Could you check a few things on this drawing? It's one solid part, dimensions in mm from its lowest x, y, z. A direction names the side the tool comes from. Round coordinates to 2 decimals unless told otherwise and drop trailing zeros. Loops run counter-clockwise (first coordinate to the right, second up) from the corner with the lowest first, then second, coordinate; pieces in that order, holes last. Notation, with made-up numbers: M 29.5,-14 L 76.5,-14 A14 ccw 76.5,12 Z; hole C 62,24 d3. An arc over 180 degrees is marked long. Answer as a JSON object with one key per item and string values.
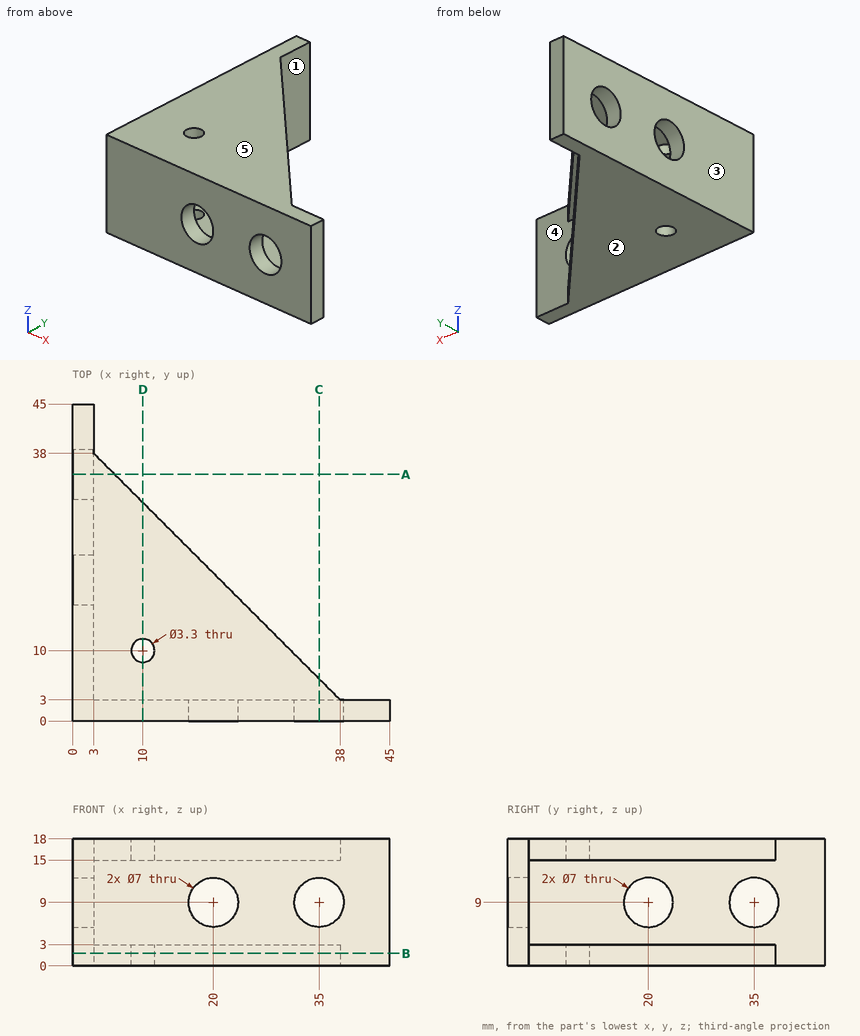
Item 1: Please list where these lines run through material, in increasing order: probe 1 along X at (y, z) = (1.9, 9); probe 2 along Z at (x, y) = (33, 4); probe 3 along Z at (x, y) = (1, 35). Write a range as from..to.
Resolved:
{"probe 1": "0..16.5, 23.5..31.5, 38.5..45", "probe 2": "0..3, 15..18", "probe 3": "0..5.5, 12.5..18"}
Item 2: I'm going to push flat-ended pins straight in: pin 1 Ø3 at (x, z) = (29, 11) entering from +Y; pin 2 Ø5 at (y, z) = (11.5, 2.5) entering from +X. Where does each tip first touch, or does it pass through?
Resolved:
{"pin 1": "y = 3", "pin 2": "x = 32"}
Item 3: I want a section at B-B, the plane z = 1.75. Please give me the cut outline in (x, y).
Resolved:
{"outline": "M 0,0 L 45,0 L 45,3 L 38,3 L 3,38 L 3,45 L 0,45 Z; hole C 10,10 d3.3"}
Item 4: I want a section at A-A, the plane y = 35. Please give me the cut outline in (x, z), then the cut area to 3 significant figures.
Resolved:
{"outline": "M 0,0 L 6,0 L 6,3 L 3,3 L 3,5.5 L 0,5.5 Z; M 0,12.5 L 3,12.5 L 3,15 L 6,15 L 6,18 L 0,18 Z", "area": "51.0 mm²"}
Item 5: On a 3-axis mill with a long thin cutter (end or side, diameter ignored), from which of +Z, -Z, +X, -X, +Y, -Y can I reach the whole of each face in a straight line? I mean the marked faces 1 and 2. Say none if no direction works.
Resolved:
{"face 1": "+X, +Y", "face 2": "-Z, +X, -X, +Y, -Y"}
Item 6: If we mould it in two halves opening along Z, with no side actions, what happens to the marked faces 3, 4 and 5? For each: pulls with the +Z half, pulls with the -Z half, needs draft (parallel to the pull), parting line crosses it, or undercut.
Resolved:
{"face 3": "needs draft", "face 4": "undercut", "face 5": "pulls with the +Z half"}
Item 7: I want a section at D-D, the plane x = 10. Please give me the cut outline in (y, z).
Resolved:
{"outline": "M 0,0 L 8.35,0 L 8.35,3 L 3,3 L 3,15 L 8.35,15 L 8.35,18 L 0,18 Z; M 11.65,0 L 31,0 L 31,3 L 11.65,3 Z; M 11.65,15 L 31,15 L 31,18 L 11.65,18 Z"}
